```python
from build123d import *

# Parameters (mm, degrees)
BOSS_EXTRUDE1_DEPTH = 69.85
SKETCH2_W           = 50.8
SKETCH2_H           = 44.45
BOSS_EXTRUDE2_DEPTH = 57.15
SKETCH3_W           = 6.35
SKETCH3_H           = 38.023239414
BOSS_EXTRUDE3_DEPTH = 6.35


with BuildPart() as part:
    # Sketch1 → Boss-Extrude1 (new body)
    with BuildSketch(Plane(origin=(0, 0, 0), x_dir=(1, 0, 0), z_dir=(0, 1, 0))):
        Polygon((0, 0), (38.1, 0), (38.1, 50.8), (12.7, 50.8), (0, 38.1), align=None)
    extrude(amount=BOSS_EXTRUDE1_DEPTH)

    # Sketch2 → Boss-Extrude2 (add)
    with BuildSketch(Plane(origin=(38.1, 0, 0), x_dir=(0, 0, -1), z_dir=(1, 0, 0))):
        with Locations((25.4, 22.225)):
            Rectangle(SKETCH2_W, SKETCH2_H)
    extrude(amount=BOSS_EXTRUDE2_DEPTH)

    # Sketch3 → Boss-Extrude3 (add)
    with BuildSketch(Plane(origin=(0, 0, 0), x_dir=(-1, 0, 0), z_dir=(0, -1, 0))):
        with Locations((-28.575, 25.024461833)):
            Rectangle(SKETCH3_W, SKETCH3_H)
        with Locations((-41.275, 25.024461833)):
            Rectangle(SKETCH3_W, SKETCH3_H)
        with Locations((-53.975, 25.024461833)):
            Rectangle(SKETCH3_W, SKETCH3_H)
        with Locations((-66.675, 25.024461833)):
            Rectangle(SKETCH3_W, SKETCH3_H)
        with Locations((-79.375, 25.024461833)):
            Rectangle(SKETCH3_W, SKETCH3_H)
    extrude(amount=BOSS_EXTRUDE3_DEPTH)


solid = part.part
```
Work out the finished part from the listing and answer in its coordinate system (mm). A direction names the side the tool comes from. Round coordinates to 2 decimals unless told otherwise and drop trailing zeros. Loops run counter-clockwise (first coordinate to the right, second up) from the corner with the lowest first, then second, coordinate; pieces in that order, holes last. Notation, with made-up numbers: M -33,27.5 L 15,27.5 A20 cw 15,57.5 Z; hole C 23,62.25 d2. An arc over 180 degrees is marked long. One line per question, with ' | ' between items.
Q1. Each of these flat-tipped pins is pushed along its axis until it touches: pin 1 Ø3 at (y, z) = (-2.5, -29.5) entering from +X; pin 2 Ø3 at (x, y) = (68, -4.5) entering from +Z; pin 3 Ø6 at (x, z) = (34.5, -12) entering from -Y; pin 4 Ø2 at (y, z) = (55, -13) entering from +X. Where does it stop, or does it pass through?
Conclusion:
pin 1: stops at x = 82.55 | pin 2: stops at z = -6.01 | pin 3: stops at y = -6.35 | pin 4: stops at x = 38.1
Q2. Find section A-A, the plane x = 65.5. Give the vertices of the cut face in (y, z), then the cut area to 3 significant figures.
Conclusion:
outline: M -6.35,-44.04 L 0,-44.04 L 0,-50.8 L 44.45,-50.8 L 44.45,0 L 0,0 L 0,-6.01 L -6.35,-6.01 Z | area: 2,500 mm2
Q3. A tool of negligible diameter and unlimited length cuts with its end or side. For faces 1 (the flat face through (44.45, -3, -25)), 2 (the flat face through (67, -3, -44.036)), 3 (the flat face through (41, -3, -6.013)), 4 (the flat face through (29, -6.35, -25)), 5 (the flat face through (0, 34, -19)), from which of +Z, -Z, +X, -X, +Y, -Y can it reach the whole face along a straight path? Write none if from no direction.
Conclusion:
face 1: +Z, -Z, -Y | face 2: -Z, +X, -X, -Y | face 3: +Z, +X, -X, -Y | face 4: +Z, -Z, +X, -X, -Y | face 5: +Z, -Z, -X, +Y, -Y
Q4. Find section D-D, the plane z = -32. Give the vertices of the cut face in (x, y).
Conclusion:
outline: M 0,0 L 25.4,0 L 25.4,-6.35 L 31.75,-6.35 L 31.75,0 L 38.1,0 L 38.1,-6.35 L 44.45,-6.35 L 44.45,0 L 50.8,0 L 50.8,-6.35 L 57.15,-6.35 L 57.15,0 L 63.5,0 L 63.5,-6.35 L 69.85,-6.35 L 69.85,0 L 76.2,0 L 76.2,-6.35 L 82.55,-6.35 L 82.55,0 L 95.25,0 L 95.25,44.45 L 38.1,44.45 L 38.1,69.85 L 0,69.85 Z
Q5. Find section C-C, the plane y = 55.5. Give the vertices of the cut face in (x, z), then the cut area to 3 significant figures.
Conclusion:
outline: M 0,-38.1 L 12.7,-50.8 L 38.1,-50.8 L 38.1,0 L 0,0 Z | area: 1,850 mm2
Q6. Consider line 1 along X through (y, z) = (-2.5, -25); line 2 along Y through (x, z) = (10.5, -40.5); line 3 along Y through (x, z) = (73, -27). Determine where each line is inside the solid, lowest interval first. Write a range as from..to.
Conclusion:
line 1: x = 25.4..31.75, 38.1..44.45, 50.8..57.15, 63.5..69.85, 76.2..82.55 | line 2: y = 0..69.85 | line 3: y = 0..44.45
Q7. The mould has two halves that part along X. Classify faces 6 (the flat face through (6.4, 34.4, -44.5)), 7 (the flat face through (38.1, -3, -25)), 8 (the flat face through (53, 27, -50.8)): +X half, -X half, draft (parallel to the pull), parting line (faces both ways), or undercut.
Conclusion:
face 6: -X half | face 7: undercut | face 8: draft
Q8. Find section B-B, the plane z = -40. Give the vertices of the cut face in (x, y), then the cut area to 3 significant figures.
Conclusion:
outline: M 1.9,0 L 25.4,0 L 25.4,-6.35 L 31.75,-6.35 L 31.75,0 L 38.1,0 L 38.1,-6.35 L 44.45,-6.35 L 44.45,0 L 50.8,0 L 50.8,-6.35 L 57.15,-6.35 L 57.15,0 L 63.5,0 L 63.5,-6.35 L 69.85,-6.35 L 69.85,0 L 76.2,0 L 76.2,-6.35 L 82.55,-6.35 L 82.55,0 L 95.25,0 L 95.25,44.45 L 38.1,44.45 L 38.1,69.85 L 1.9,69.85 Z | area: 5,270 mm2
